Work out the finished part from the listing and answer in its coordinate system (mm). Coordinates: 2 decimals unless noted, no trailing zeros.
1. Flat-ended cylindrical pins translate along their axes: pin 1 Ø10.5 at (x, y) = (0, 0) entering from -Z; pin 2 Ø2 at (y, z) = (2, 2) entering from -X; pin 3 Ø3 at (y, z) = (-4.5, 4) entering from +X; pin 4 Ø4 at (x, z) = (4.5, 4.5) entering from -Y. Find the tip coordinate at first contact, or state that the pin passes through.
2. Find the intervals of material crossed by probe 1 along Y at (x, z) = (0, 3.5); probe 2 along X at (y, z) = (6, 6.5); probe 3 along Y at (x, z) = (3, 4.25), in increasing order.
3. The part is cut by section A-A, the plane z = 3. Count the separate pieces of the cut face and the enclosed holes in it, then the cut area to 3 significant figures.
```python
from build123d import *

# Parameters (mm, degrees)
SKETCH_R           = 9
SKETCH_R_2         = 0.8
SKETCH_R_3         = 4
EXTRUDE_DEPTH      = 8
CHAMFER_1_SIZE2    = 0.75
CHAMFER_1_SIZE     = 2
CHAMFER_2_SIZE2    = 0.75
CHAMFER_2_SIZE     = 2
CHAMFER_3_SIZE2    = 0.75
CHAMFER_3_SIZE     = 2
CHAMFER_4_SIZE2    = 0.75
CHAMFER_4_SIZE     = 2
CHAMFER_5_SIZE2    = 0.75
CHAMFER_5_SIZE     = 2
CHAMFER_6_SIZE2    = 0.75
CHAMFER_6_SIZE     = 2
CHAMFER_7_SIZE2    = 0.75
CHAMFER_7_SIZE     = 2
CHAMFER_8_SIZE2    = 0.75
CHAMFER_8_SIZE     = 2
CHAMFER_9_SIZE2    = 0.75
CHAMFER_9_SIZE     = 2
CHAMFER_10_SIZE2   = 0.75
CHAMFER_10_SIZE    = 2
CHAMFER_11_SIZE2   = 0.75
CHAMFER_11_SIZE    = 2
CHAMFER_12_SIZE2   = 0.75
CHAMFER_12_SIZE    = 2
CHAMFER_13_SIZE2   = 0.75
CHAMFER_13_SIZE    = 2
CHAMFER001_1_SIZE2 = 0.75
CHAMFER001_1_SIZE  = 0.5
CHAMFER001_2_SIZE2 = 0.75
CHAMFER001_2_SIZE  = 0.5


with BuildPart() as part:
    # Sketch → Extrude (new body)
    with BuildSketch(Plane.XY):
        Circle(SKETCH_R)
        with Locations((-3.020701, 5.755464)):
            Circle(SKETCH_R_2, mode=Mode.SUBTRACT)
        with Locations((-5.349395, 3.692421)):
            Circle(SKETCH_R_2, mode=Mode.SUBTRACT)
        with Locations((-6.452608, 0.783488)):
            Circle(SKETCH_R_2, mode=Mode.SUBTRACT)
        with Locations((-6.077606, -2.304932)):
            Circle(SKETCH_R_2, mode=Mode.SUBTRACT)
        with Locations((-4.310297, -4.86532)):
            Circle(SKETCH_R_2, mode=Mode.SUBTRACT)
        with Locations((-1.555552, -6.311122)):
            Circle(SKETCH_R_2, mode=Mode.SUBTRACT)
        with Locations((1.555552, -6.311122)):
            Circle(SKETCH_R_2, mode=Mode.SUBTRACT)
        with Locations((4.310297, -4.86532)):
            Circle(SKETCH_R_2, mode=Mode.SUBTRACT)
        with Locations((6.077606, -2.304932)):
            Circle(SKETCH_R_2, mode=Mode.SUBTRACT)
        with Locations((6.452608, 0.783488)):
            Circle(SKETCH_R_2, mode=Mode.SUBTRACT)
        with Locations((5.349395, 3.692421)):
            Circle(SKETCH_R_2, mode=Mode.SUBTRACT)
        with Locations((3.020701, 5.755464)):
            Circle(SKETCH_R_2, mode=Mode.SUBTRACT)
        with Locations((0, 6.5)):
            Circle(SKETCH_R_2, mode=Mode.SUBTRACT)
        Circle(SKETCH_R_3, mode=Mode.SUBTRACT)
    extrude(amount=EXTRUDE_DEPTH)

    # Chamfer 1
    chamfer_1_edges = [part.edges().sort_by_distance(p)[0] for p in [
        (-3.820701, 5.755464, 0),
    ]]
    chamfer_1_side = part.faces().sort_by_distance((-3.820701, 5.755464, 4))[0]
    chamfer(chamfer_1_edges, length=CHAMFER_1_SIZE, length2=CHAMFER_1_SIZE2, reference=chamfer_1_side)

    # Chamfer 2
    chamfer_2_edges = [part.edges().sort_by_distance(p)[0] for p in [
        (-5.110297, -4.86532, 0),
    ]]
    chamfer_2_side = part.faces().sort_by_distance((-5.110297, -4.86532, 4))[0]
    chamfer(chamfer_2_edges, length=CHAMFER_2_SIZE, length2=CHAMFER_2_SIZE2, reference=chamfer_2_side)

    # Chamfer 3
    chamfer_3_edges = [part.edges().sort_by_distance(p)[0] for p in [
        (3.510297, -4.86532, 0),
    ]]
    chamfer_3_side = part.faces().sort_by_distance((3.510297, -4.86532, 4))[0]
    chamfer(chamfer_3_edges, length=CHAMFER_3_SIZE, length2=CHAMFER_3_SIZE2, reference=chamfer_3_side)

    # Chamfer 4
    chamfer_4_edges = [part.edges().sort_by_distance(p)[0] for p in [
        (4.549395, 3.692421, 0),
    ]]
    chamfer_4_side = part.faces().sort_by_distance((4.549395, 3.692421, 4))[0]
    chamfer(chamfer_4_edges, length=CHAMFER_4_SIZE, length2=CHAMFER_4_SIZE2, reference=chamfer_4_side)

    # Chamfer 5
    chamfer_5_edges = [part.edges().sort_by_distance(p)[0] for p in [
        (-6.877606, -2.304932, 0),
    ]]
    chamfer_5_side = part.faces().sort_by_distance((-6.877606, -2.304932, 4))[0]
    chamfer(chamfer_5_edges, length=CHAMFER_5_SIZE, length2=CHAMFER_5_SIZE2, reference=chamfer_5_side)

    # Chamfer 6
    chamfer_6_edges = [part.edges().sort_by_distance(p)[0] for p in [
        (-2.355552, -6.311122, 0),
    ]]
    chamfer_6_side = part.faces().sort_by_distance((-2.355552, -6.311122, 4))[0]
    chamfer(chamfer_6_edges, length=CHAMFER_6_SIZE, length2=CHAMFER_6_SIZE2, reference=chamfer_6_side)

    # Chamfer 7
    chamfer_7_edges = [part.edges().sort_by_distance(p)[0] for p in [
        (5.277606, -2.304932, 0),
    ]]
    chamfer_7_side = part.faces().sort_by_distance((5.277606, -2.304932, 4))[0]
    chamfer(chamfer_7_edges, length=CHAMFER_7_SIZE, length2=CHAMFER_7_SIZE2, reference=chamfer_7_side)

    # Chamfer 8
    chamfer_8_edges = [part.edges().sort_by_distance(p)[0] for p in [
        (-7.252608, 0.783488, 0),
    ]]
    chamfer_8_side = part.faces().sort_by_distance((-7.252608, 0.783488, 4))[0]
    chamfer(chamfer_8_edges, length=CHAMFER_8_SIZE, length2=CHAMFER_8_SIZE2, reference=chamfer_8_side)

    # Chamfer 9
    chamfer_9_edges = [part.edges().sort_by_distance(p)[0] for p in [
        (0.755552, -6.311122, 0),
    ]]
    chamfer_9_side = part.faces().sort_by_distance((0.755552, -6.311122, 4))[0]
    chamfer(chamfer_9_edges, length=CHAMFER_9_SIZE, length2=CHAMFER_9_SIZE2, reference=chamfer_9_side)

    # Chamfer 10
    chamfer_10_edges = [part.edges().sort_by_distance(p)[0] for p in [
        (5.652608, 0.783488, 0),
    ]]
    chamfer_10_side = part.faces().sort_by_distance((5.652608, 0.783488, 4))[0]
    chamfer(chamfer_10_edges, length=CHAMFER_10_SIZE, length2=CHAMFER_10_SIZE2, reference=chamfer_10_side)

    # Chamfer 11
    chamfer_11_edges = [part.edges().sort_by_distance(p)[0] for p in [
        (-0.8, 6.5, 0),
    ]]
    chamfer_11_side = part.faces().sort_by_distance((-0.8, 6.5, 4))[0]
    chamfer(chamfer_11_edges, length=CHAMFER_11_SIZE, length2=CHAMFER_11_SIZE2, reference=chamfer_11_side)

    # Chamfer 12
    chamfer_12_edges = [part.edges().sort_by_distance(p)[0] for p in [
        (-6.149395, 3.692421, 0),
    ]]
    chamfer_12_side = part.faces().sort_by_distance((-6.149395, 3.692421, 4))[0]
    chamfer(chamfer_12_edges, length=CHAMFER_12_SIZE, length2=CHAMFER_12_SIZE2, reference=chamfer_12_side)

    # Chamfer 13
    chamfer_13_edges = [part.edges().sort_by_distance(p)[0] for p in [
        (2.220701, 5.755464, 0),
    ]]
    chamfer_13_side = part.faces().sort_by_distance((2.220701, 5.755464, 4))[0]
    chamfer(chamfer_13_edges, length=CHAMFER_13_SIZE, length2=CHAMFER_13_SIZE2, reference=chamfer_13_side)

    # Chamfer001 1
    chamfer001_1_edges = [part.edges().sort_by_distance(p)[0] for p in [
        (-6.149395, 3.692421, 8),
        (-0.8, 6.5, 8),
        (5.652608, 0.783488, 8),
        (0.755552, -6.311122, 8),
        (-7.252608, 0.783488, 8),
        (5.277606, -2.304932, 8),
        (-2.355552, -6.311122, 8),
        (-6.877606, -2.304932, 8),
        (4.549395, 3.692421, 8),
        (3.510297, -4.86532, 8),
        (-5.110297, -4.86532, 8),
        (-3.820701, 5.755464, 8),
    ]]
    chamfer001_1_side = part.faces().sort_by_distance((-8.745442, 0, 8))[0]
    chamfer(chamfer001_1_edges, length=CHAMFER001_1_SIZE, length2=CHAMFER001_1_SIZE2, reference=chamfer001_1_side)

    # Chamfer001 2
    chamfer001_2_edges = [part.edges().sort_by_distance(p)[0] for p in [
        (2.220701, 5.755464, 8),
    ]]
    chamfer001_2_side = part.faces().sort_by_distance((2.220701, 5.755464, 5))[0]
    chamfer(chamfer001_2_edges, length=CHAMFER001_2_SIZE, length2=CHAMFER001_2_SIZE2, reference=chamfer001_2_side)


solid = part.part
```
Geometry says:
1. pin 1: stops at z = 0
1. pin 2: stops at x = -8.94
1. pin 3: stops at x = 8.49
1. pin 4: stops at y = -8.65
2. probe 1: y = -9 to -4, 4 to 5.7, 7.3 to 9
2. probe 2: x = -6.71 to -3.78, -2.26 to -0.62, 0.62 to 2.26, 3.78 to 6.71
2. probe 3: y = -8.49 to -2.65, 2.65 to 4.96, 6.56 to 8.49
3. separate pieces: 1
3. enclosed holes: 14
3. area: 178 mm2
